Design review of the part built by this model. Coordinates are the model's own, in mm. Face numbers are marked on the shaded views. A direction names the side the tool comes from. Give positions to 0.01 mm unless a question says otherwise; leave off trailing zeros. Loops run counter-clockwise (first coordinate to the right, second up) from the corner with the lowest first, then second, coordinate; pieces in that order, holes last. Notation, with made-up numbers: (49.25, -11) - (98.25, -11) arc R12 ccw to (98.25, 0) - close; hole circle Ø9 at (29.25, 26.5). An arc over 180 degrees is marked (long way). One line per item, written item: value. Start each with the question number.
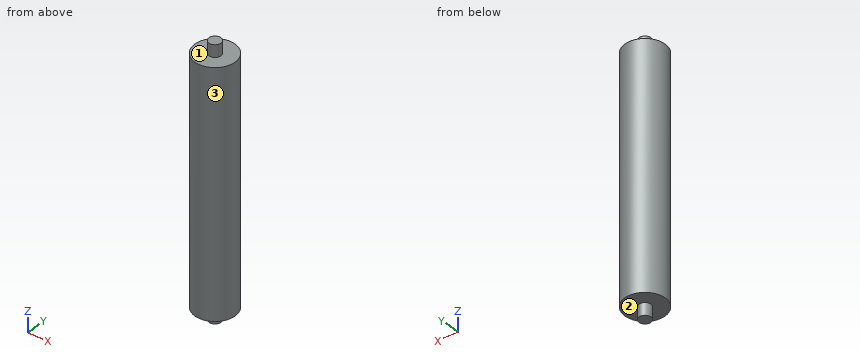
```python
from build123d import *

# Parameters (mm, degrees)
SKETCH1_R           = 25
BOSS_EXTRUDE1_DEPTH = 150
SHELL1_T            = 5
SKETCH2_R           = 7.5
BOSS_EXTRUDE2_DEPTH = 15


with BuildPart() as part:
    # Sketch1 → Boss-Extrude1 (new, symmetric)
    with BuildSketch(Plane.XY):
        Circle(SKETCH1_R)
    extrude(amount=BOSS_EXTRUDE1_DEPTH, both=True)

    # Shell1 (no face opened: a closed hollow body)
    add(offset(amount=-SHELL1_T, mode=Mode.PRIVATE), mode=Mode.SUBTRACT)

    # Sketch2 → Boss-Extrude2 (add)
    with BuildSketch(Plane.XY.offset(150)):
        Circle(SKETCH2_R)
    boss_extrude2 = extrude(amount=BOSS_EXTRUDE2_DEPTH)

    # Mirror1: Boss-Extrude2 across plane
    add(boss_extrude2.mirror(Plane.XY))


solid = part.part
```
(1) Take a section at A-A on x = 0. State the section outline as (y, z) points, and give its area (3 significant figures).
(2) Take a section at D-D on x = -16. State the section outline as (y, z) points.
(3) Machinability: for the marked faces 1, 2 and 3, which of the approach directions +Z, -Z, +X, -X, +Y, -Y give a long, thin tool a straight path to every point of the face, cutting with its end or side? Answer none if there is none.
(4) To check wall thickness, follow L1, parallel to Y at x = 0, z = -70; L2, parallel to Z at x = -17.5, y = 4; L3, parallel to X at y = -1, z = -125. State the ranges of each line that lie inside material, in increasing order. Write a range as from..to.
(5) For pin 1 Ø10 at (x, z) = (5.5, 108.5) entering from +Y (3 decimals); pin 2 Ø12 at (x, y) = (14.5, 9.5) entering from -Z; pin 3 Ø10 at (x, z) = (-19.5, 55.5) entering from +Y, all flat-tipped, find the tip position at first contact; note any pin that passes through.
(6) Take a section at C-C on z = -33.5. State the section outline as (x, y) points.
Here are the results:
1. outline: (-25, -150) - (-7.5, -150) - (-7.5, -165) - (7.5, -165) - (7.5, -150) - (25, -150) - (25, 150) - (7.5, 150) - (7.5, 165) - (-7.5, 165) - (-7.5, 150) - (-25, 150) - close; hole (-20, -145) - (20, -145) - (20, 145) - (-20, 145) - close
1. area: 3,850 mm²
2. outline: (-19.21, -150) - (19.21, -150) - (19.21, 150) - (-19.21, 150) - close; hole (-12, -145) - (12, -145) - (12, 145) - (-12, 145) - close
3. face 1: +Z
3. face 2: -Z
3. face 3: +Z, -Z
4. L1: -25..-20, 20..25
4. L2: -150..-145, 145..150
4. L3: -24.98..-19.97, 19.97..24.98
5. pin 1: y = 24.995
5. pin 2: z = -150
5. pin 3: y = 20.37
6. outline: circle Ø50 at (0, 0); hole circle Ø40 at (0, 0)
